Can you work these out from the model? Positions are in its coordinate system, mm. A direction names the side the tool comes from. Give positions to 0.01 mm unless a question says otherwise; leave off trailing zeros. Write each loop counter-clockwise with the first axis right and the second up, starting at its lowest first coordinate (ties: lowest second). Pieces come first, ordered by that corner, then holes. Notation, with made-up numbers: (-1.75, -9.5) - (36.25, -9.5) arc R12 ccw to (36.25, -1.5) - close; hole circle Ø10 at (-13.75, 88). An arc over 180 degrees is marked (long way). Use a Markdown table: item, result. Add a question column.
```python
from build123d import *

# Parameters (mm, degrees)
EXTRUDE_1_DEPTH     = 4
SKETCH_4_OUTSIDE_W  = 19.022
SKETCH_4_OUTSIDE_H  = 13.522
SKETCH_4_OUTSIDE_R  = 4
CUT_EXTRUDE_1_DEPTH = 2.2
CUT_EXTRUDE_2_DEPTH = 6.8


with BuildPart() as part:
    # Эскиз1 → Бобышка-Вытянуть1 (new body, symmetric)
    with BuildSketch(Plane.XY):
        Polygon((4, 0), (-4, 0), (-4, -2.2), (-6.75, -2.2), (-6.75, -8), (6.75, -8), (6.75, -2.2), (4, -2.2), align=None)
    extrude(amount=EXTRUDE_1_DEPTH, both=True)

    # Эскиз3 → Отверстие обработанное метчиком M51 (revolve, cut)
    with BuildSketch(Plane(origin=(0, 0, 0), x_dir=(0, 0, 1), z_dir=(1, 0, 0))):
        Polygon((0, 0), (0, 8), (3.1, 8), (2.1, 7), (2.1, 1), (3.1, 0), align=None)
    revolve(axis=Axis((0, 6.35, 0), (0, -1, 0)), mode=Mode.SUBTRACT)

    # Эскиз4 outside → Вырез-Вытянуть1 (cut)
    with BuildSketch(Plane(origin=(0, 0, 0), x_dir=(1, 0, 0), z_dir=(0, 1, 0))):
        Rectangle(SKETCH_4_OUTSIDE_W, SKETCH_4_OUTSIDE_H)
        with Locations(Location((0, 0, 0), (0, 0, 270))):  # turned: the seam where the file's is
            Circle(SKETCH_4_OUTSIDE_R, mode=Mode.SUBTRACT)
    extrude(amount=-CUT_EXTRUDE_1_DEPTH, mode=Mode.SUBTRACT)

    # Эскиз5 → Вырез-Вытянуть2 (cut, through all)
    with BuildSketch(Plane(origin=(0, -2.2, 0), x_dir=(1, 0, 0), z_dir=(0, 1, 0))):
        with BuildLine():
            Line((-6.75, 0), (-6.75, 4))
            Line((-6.75, 4), (-5.437140793, 4))
            ThreePointArc((-5.437140793, 4), (-6.413392252, 2.104970267), (-6.75, 0))
        make_face()
        with BuildLine():
            Line((6.75, 0), (6.75, -4))
            Line((6.75, -4), (5.437140793, -4))
            ThreePointArc((5.437140793, -4), (6.413392252, -2.104970267), (6.75, 0))
        make_face()
    extrude(amount=-CUT_EXTRUDE_2_DEPTH, mode=Mode.SUBTRACT)

    # Вырез-По траектории1: sweep along a path in Эскиз7
    with BuildLine(Plane.XZ.offset(8)) as sweep_1_path:
        Line((0, 6.75), (-6.75, 6.75))
        Line((-6.75, 6.75), (-6.75, 0))
        ThreePointArc((-6.75, 0), (-4.772970773, -4.772970773), (0, -6.75))
        Line((0, -6.75), (6.75, -6.75))
        Line((6.75, -6.75), (6.75, 0))
        ThreePointArc((6.75, 0), (4.772970773, 4.772970773), (0, 6.75))
    # Эскиз6 → Вырез-По траектории1 (sweep, cut)
    with BuildSketch(Plane.XY.offset(4)):
        Polygon((-6.75, -4.7), (-6.75, -8), (-4, -8), align=None)
    sweep(path=sweep_1_path.line, transition=Transition.RIGHT, mode=Mode.SUBTRACT)


solid = part.part
```
Q1. If I drill on probe 1 along X at (y, z) = (-2.95, 0); probe 2 along X at (y, z) = (-4.8, 0); probe 3 along Z at (x, y) = (2, -7.25), over which ranges is the centre line in solid material (lowest first)? Write a range as [from, to].
Q2. Suppose I cut it at A-A (y = -5.5). Please give me the cut outline in (x, z).
Q3. I'm going to push flat-ended pins straight in: P1, Ø2, axis at y = -6, z = -1, coming from the -X side; P2, Ø3.5, axis at x = 0, z = 0, coming from the -Y side. Where does each tip first touch, or does it pass through?
Q4. If we mould it in two halves opening along X, with no side actions, what happens to faces 1 (the cylindrical face through (-0.631, -3.958, 2.003)), 2 (the conical face through (4.64, -6.69, 2.1)), 3 (the flat face through (-5, -2.2, 0)), 4 (the flat face through (-6.75, -3, 2))? For each: released by +X, released by -X, zero draft, split by the parting line, or undercut.
Q5. Suppose I cut it at B-B (y = -0.5). Please give me the cut outline in (x, z).
Q6. On a 3-axis mill with a long thin cutter (end or side, diameter ignored), from which of +Z, -Z, +X, -X, +Y, -Y can I reach the whole of each face in a straight line? I mean faces 5 (the flat face through (-5.36, -6.37, 1.97)), 6 (the cylindrical face through (-3.905, -1.085, -0.867)). Say none if no direction works.
Derived:
| question | item | result |
|---|---|---|
| 1 | probe 1 | [-6.75, -2.1], [2.1, 6.75] |
| 1 | probe 2 | [-6.67, -2.1], [2.1, 6.67] |
| 1 | probe 3 | [-4, -1.23], [1.23, 4] |
| 2 | outline | (-6.08, 0) arc R6.08 ccw to (-4.58, -4) - (6.08, -4) - (6.08, 0) arc R6.08 ccw to (4.58, 4) - (-6.08, 4) - close; hole circle Ø4.2 at (0, 0) |
| 3 | P1 | x = -6.43 |
| 3 | P2 | through |
| 4 | face 1 | undercut |
| 4 | face 2 | released by +X |
| 4 | face 3 | zero draft |
| 4 | face 4 | released by -X |
| 5 | outline | circle Ø8 at (0, 0); hole circle Ø5.2 at (0, 0) |
| 6 | face 5 | +Z, -Z, -X, -Y |
| 6 | face 6 | +Y |
